Check sheet for the modelled part. Datum: model origin and axes. Units: mm. A direction names the side the tool comes from. Coordinates: 2 decimals unless noted, no trailing zeros. Write each loop counter-clockwise with the first axis right and the second up, starting at its lowest first coordinate (ties: lowest second). Pieces come first, ordered by that corner, then holes. Notation, with made-up numbers: (-15, 40.5) - (7, 40.5) arc R34 ccw to (7, 77.5) - close; hole circle Ø4 at (-33, -11.75). An arc over 180 degrees is marked (long way). Write each question's results on one line, items separated by ' | '.
from build123d import *

# Parameters (mm, degrees)
SKETCH_1_W          = 39.8
SKETCH_1_H          = 7.8
EXTRUDE_1_DEPTH     = 3.2
SKETCH_2_R          = 2.5
CUT_EXTRUDE_1_DEPTH = 1.8


with BuildPart() as part:
    # Эскиз1 → Бобышка-Вытянуть1 (new body)
    with BuildSketch(Plane(origin=(0, 0, 0), x_dir=(1, 0, 0), z_dir=(0, 1, 0))):
        Rectangle(SKETCH_1_W, SKETCH_1_H)
    extrude(amount=EXTRUDE_1_DEPTH)

    # Эскиз2 → Вырез-Вытянуть1 (cut)
    with BuildSketch(Plane.XZ):
        with Locations(Location((16, 0, 0), (0, 0, 270))):
            Circle(SKETCH_2_R)
        with Locations(Location((8.126, 0, 0), (0, 0, 270))):
            Circle(SKETCH_2_R)
        with Locations(Location((0.252, 0, 0), (0, 0, 270))):
            Circle(SKETCH_2_R)
        with Locations(Location((-7.622, 0, 0), (0, 0, 270))):
            Circle(SKETCH_2_R)
        with Locations(Location((-15.496, 0, 0), (0, 0, 270))):
            Circle(SKETCH_2_R)
    extrude(amount=-CUT_EXTRUDE_1_DEPTH, mode=Mode.SUBTRACT)


solid = part.part
1. Access from +Z, -Z, +X, -X, +Y, -Y to the whole of each face (thin tool, end or side, straight path). Record for faces 5 (the flat face through (19.9, 2, 0)), 6 (the flat face through (-8, 1.8, 0)).
Values follow:
face 5: +Z, -Z, +X, +Y, -Y | face 6: -Y
2. Sectioned sample at C-C (x = 16). Record the cut outline in (y, z).
Values follow:
outline: (0, -3.9) - (3.2, -3.9) - (3.2, 3.9) - (0, 3.9) - (0, 2.5) - (1.8, 2.5) - (1.8, -2.5) - (0, -2.5) - close
3. Sectioned sample at A-A (z = 0). Record the cut outline in (x, y), then the cut area to 3 significant figures.
Values follow:
outline: (-19.9, 0) - (-18, 0) - (-18, 1.8) - (-13, 1.8) - (-13, 0) - (-10.12, 0) - (-10.12, 1.8) - (-5.12, 1.8) - (-5.12, 0) - (-2.25, 0) - (-2.25, 1.8) - (2.75, 1.8) - (2.75, 0) - (5.63, 0) - (5.63, 1.8) - (10.63, 1.8) - (10.63, 0) - (13.5, 0) - (13.5, 1.8) - (18.5, 1.8) - (18.5, 0) - (19.9, 0) - (19.9, 3.2) - (-19.9, 3.2) - close | area: 82.4 mm^2
4. Sectioned sample at D-D (x = 8.5). Record the cut outline in (y, z), then the cut area to 3 significant figures.
Values follow:
outline: (0, -3.9) - (3.2, -3.9) - (3.2, 3.9) - (0, 3.9) - (0, 2.47) - (1.8, 2.47) - (1.8, -2.47) - (0, -2.47) - close | area: 16.1 mm^2
5. Go/stop test with a flat-tipped pin: pin 1 (1.5 mm diameter, centred on x = 16.5, z = -0.5, fed in from -Y). Record where the tip stops, or that it passes through.
Values follow:
pin 1: stops at y = 1.8
6. Material ranges on L1, parallel to X at y = 0.65, z = 0; L2, parallel to X at y = 1.05, z = -2; L3, parallel to Z at x = -8, y = 1.5, recorded low to high. Write a range as [from, to].
Values follow:
L1: x = [-19.9, -18], [-13, -10.12], [-5.12, -2.25], [2.75, 5.63], [10.63, 13.5], [18.5, 19.9] | L2: x = [-19.9, -17], [-14, -9.12], [-6.12, -1.25], [1.75, 6.63], [9.63, 14.5], [17.5, 19.9] | L3: z = [-3.9, -2.47], [2.47, 3.9]
7. Sectioned sample at B-B (y = 0.75). Record the cut outline in (x, z), then the cut area to 3 significant figures.
Values follow:
outline: (-19.9, -3.9) - (19.9, -3.9) - (19.9, 3.9) - (-19.9, 3.9) - close; hole circle Ø5 at (-15.5, 0); hole circle Ø5 at (-7.62, 0); hole circle Ø5 at (0.25, 0); hole circle Ø5 at (8.13, 0); hole circle Ø5 at (16, 0) | area: 212 mm^2
8. Draft check along Z on faces 1 (the cylindrical face through (10.605, 0.887, 0.325)), 2 (the flat face through (0, 2, 3.9)), 3 (the cylindrical face through (-13.017, 0.887, 0.325)), 4 (the flat face through (0, 3.2, 0)). Enter one of: pulls with the +Z half, pulls with the -Z half, needs draft (parallel to the pull), parting line crosses it, or undercut.
Values follow:
face 1: undercut | face 2: pulls with the +Z half | face 3: undercut | face 4: needs draft
